Check sheet for the modelled part. Datum: model origin and axes. Units: mm. A direction names the side the tool comes from. Give positions to 0.01 mm unless a question says otherwise; leave off trailing zeros. Write each loop counter-clockwise with the first axis right and the second up, starting at its lowest first coordinate (ties: lowest second). Pieces come first, ordered by that corner, then holes. Notation, with made-up numbers: M 74.5,82 L 83.5,82 A24 ccw 83.5,102 Z; hole C -22,-24.5 d7. An arc over 180 degrees is marked long. One line per item, written item: value. Start each with the question number.
from build123d import *


with BuildPart() as f1:
    # F0 (on Front) → F1 (revolve)
    with BuildSketch(Plane.XZ):
        with BuildLine():
            Line((17.25, 7.861132), (17.25, 0))
            Line((17.25, 0), (46.25, 0))
            Line((46.25, 0), (49.25, 0))
            Line((49.25, 0), (49.25, 2))
            Line((49.25, 2), (46.25, 2))
            Line((46.25, 2), (46.25, 20))
            Line((46.25, 20), (19.272028, 10.697251))
            ThreePointArc((19.272028, 10.697251), (17.807264, 9.602695), (17.25, 7.861132))
        make_face()
    revolve(axis=Axis((0, 0, 5.085478), (0, 0, -1)))


solid = f1.part
1) Cross-section at D-D (z = 5). Record the boundary of the cut face in (x, y).
2) Material ranges on L1, parallel to X at y = 0, z = 3.75; L2, parallel to Y at x = 0, z = 1.5, recorded low to high. Write a range as from..to.
3) Tool access check on faces 4 (the flat face through (-15, -44, 2)), 5 (the cylindrical face through (46.976, -14.793, 1.014)). Record the directions out of +Z, -Z, +X, -X, +Y, -Y that give a thin tool (end or side, any length) a straight path to the whole face; none if there is none.
4) Cross-section at C-C (z = 13). Record the boundary of the cut face in (x, y), plus the area to 3 significant figures.
5) Gauge pin test, flat ends, axial feed: pin 1 (1.5 mm diameter, centred on x = -11, z = 17.5, fed in from -Y); pin 2 (8 mm diameter, centred on x = 1.5, z = 3, fed in from -Y); pin 3 (2 mm diameter, centred on y = -6.5, z = 8, fed in from +X). Record the tip position at first contact, or that the pin passes through.
6) Draft check along X on faces 1 (the cylindrical face through (16.453, -5.181, 3.876)), 2 (the cylindrical face through (24.86, -39, 11.13)), 3 (the flat face through (-21, -1, 0)). Enter one of: released by +X, released by -X, zero draft, split by the parting line, or undercut.
7) Cross-section at A-A (y = 0). Record the boundary of the cut face in (x, z), plus the area to 3 significant figures.
Data:
1. outline: C 0,0 d92.5; hole C 0,0 d34.5
2. L1: x = -46.25..-17.25, 17.25..46.25
2. L2: y = -49.25..-17.25, 17.25..49.25
3. face 4: +Z
3. face 5: +Z, -Z
4. outline: C 0,0 d92.5; hole C 0,0 d51.9
4. area: 4,600 mm2
5. pin 1: stops at y = -45.1
5. pin 2: stops at y = -49.25
5. pin 3: stops at x = 45.92
6. face 1: undercut
6. face 2: split by the parting line
6. face 3: zero draft
7. outline: M -49.25,0 L -17.25,0 L -17.25,7.86 A3 ccw -19.27,10.7 L -46.25,20 L -46.25,2 L -49.25,2 Z; M 17.25,0 L 49.25,0 L 49.25,2 L 46.25,2 L 46.25,20 L 19.27,10.7 A3 ccw 17.25,7.86 Z
7. area: 880 mm2
